Input: part model. Units: mm. Frame: model coordinates. A direction names the side the tool comes from. Coordinates: 2 decimals unless noted, no trailing zeros. Write each loop counter-clockwise with the first axis right and the second up, starting at its lowest first coordinate (ties: lowest second). Pieces come first, ordered by that corner, then holes. Notation, with made-up numbers: M 88.25,89.25 L 131.25,89.25 A36 ccw 131.25,124.25 Z; hole C 36.5,-36 d8. An arc over 180 degrees is marked long. Use CSV: the item, a comma, the result in double quotes.
Autodesk Inventor part; units mm, degrees
ref_plane "YZ Plane" through (0, 0, 0) normal (1, 0, 0) x (0, 1, 0)
ref_plane "XZ Plane" through (0, 0, 0) normal (0, 1, 0) x (-1, 0, 0)
ref_plane "XY Plane" through (0, 0, 0) normal (0, 0, 1) x (1, 0, 0)
sketch "Sketch1" plane through (0, 0, 0) normal (0, 0, 1) x (1, 0, 0)
  arc A0 (20, 0) -> (-20, 0) centre (0, 0) ccw
  line L0 (-20, 0) -> (-20, -104)
  line L1 (20, 0) -> (20, -52)
  arc A1 (19.4895, -54.5451) -> (20, -52) centre (13.4, -52) ccw
  arc A2 (-20, -104) -> (-7.0525, -122.7153) centre (0, -104) ccw
  arc A3 (-7.0525, -122.7153) -> (19.963, -105.2168) centre (0, -104) ccw
  arc A4 (19.963, -105.2168) -> (12.0286, -88.0215) centre (0, -104) ccw
  arc A5 (9.4588, -78.5451) -> (12.0286, -88.0215) centre (16.84, -81.6301) ccw
  line L2 (9.4588, -78.5451) -> (19.4895, -54.5451)
  line L3 (-10, 5.5) -> (10.3, 5.5)
  line L4 (10.3, 5.5) -> (10.3, -35.5)
  line L5 (10.3, -35.5) -> (-10, -35.5)
  line L6 (-10, -35.5) -> (-10, 5.5)
  dimension "d3" = 20
  dimension "d5" = 52
  dimension "d6" = 20
  dimension "d7" = 20
  dimension "d8" = 8
  dimension "d10" = 6.6
  dimension "d11" = 24
  dimension "d17" = 20.3
  dimension "d18" = 41
  dimension "d19" = 10
  dimension "d20" = 104
  dimension "d30" = 5.5
extrude "Extrusion1" add sketch "Sketch1" along normal blind 3.3
sketch "Sketch2" plane through (0, 0, 3.3) normal (0, 0, 1) x (1, 0, 0)
  line L0 (-10, 5.5) -> (10.3, 5.5)
  line L1 (10.3, -35.5) -> (-10, -35.5)
  circle A0 centre (-5, 10) radius 1
  circle A1 centre (-5, -40.25) radius 1
  line L2 (-10, -35.5) -> (-10, 5.5)
  line L3 (10.3, 5.5) -> (10.3, -35.5)
  circle A2 centre (5, 10) radius 1
  circle A3 centre (5, -40.25) radius 1
  point P0 (0, 0)
  dimension "d31" = 2
  dimension "d32" = 2
  dimension "d34" = 4.5
  dimension "d36" = 4.75
  dimension "d65" = 5
  dimension "d66" = 10
  dimension "d67" = 5
  dimension "d68" = 10
extrude "Extrusion2" cut sketch "Sketch2" against normal blind 4.5 contours A0 | A1 | A2 | A3
sketch "Sketch3" plane through (0, 0, 3.3) normal (0, 0, 1) x (1, 0, 0)
  line L0 (-20, 0) -> (-20, -104)
  line L1 (10.3, 5.5) -> (10.3, -35.5)
  line L2 (10.3, -35.5) -> (-10, -35.5)
  line L3 (-10, -35.5) -> (-10, 5.5)
  line L4 (-10, 5.5) -> (10.3, 5.5)
  line L5 (-20, 0) -> (-20, -104)
  arc A0 (-20, -104) -> (12.0286, -88.0215) centre (0, -104) ccw
  arc A1 (9.4588, -78.5451) -> (12.0286, -88.0215) centre (16.84, -81.6301) ccw
  line L6 (9.4588, -78.5451) -> (19.4895, -54.5451)
  arc A2 (19.4895, -54.5451) -> (20, -52) centre (13.4, -52) ccw
  line L7 (20, -52) -> (20, 0)
  arc A3 (20, 0) -> (-20, 0) centre (0, 0) ccw
  line L8 (-15, -86) -> (-15, -56)
  line L9 (15, -45.2979) -> (15, -53.2979)
  line L10 (15, -53.2979) -> (4.448, -78.5451)
  line L11 (4.448, -78.5451) -> (-15, -86)
  line L12 (9.4588, -78.5451) -> (19.4895, -54.5451)
  line L13 (-15, -94.5676) -> (-15, -104)
  arc A4 (-15, -104) -> (9.0215, -92.0161) centre (0, -104) ccw
  arc A5 (-20, -104) -> (12.0286, -88.0215) centre (0, -104) ccw
  arc A6 (4.9629, -86.9153) -> (9.0215, -92.0161) centre (16.84, -81.6301) ccw
  arc A7 (9.4588, -78.5451) -> (12.0286, -88.0215) centre (16.84, -81.6301) ccw
  line L14 (4.9629, -86.9153) -> (-15, -94.5676)
  line L15 (-15, -56) -> (15, -45.2979)
  line L16 (-15, -50.6914) -> (15, -39.9893)
  line L17 (15, -39.9893) -> (15, -36.8041)
  line L18 (15, -36.8041) -> (-15, -47.5062)
  line L19 (-15, -47.5062) -> (-15, -50.6914)
  point P0 (19.8711, -53.2979)
  dimension "d45" = 5
  dimension "d46" = 5
  dimension "d48" = 8
  dimension "d49" = 18
  dimension "d52" = 5
  dimension "d54" = 3
  dimension "d56" = 30
  dimension "d57" = 8
sketch "Sketch4" plane through (0, 0, 3.3) normal (0, 0, 1) x (1, 0, 0)
  line L0 (10.3, 5.5) -> (-10, 5.5)
  line L1 (-3.6, 5.5) -> (3.6, 5.5)
  line L2 (3.6, 5.5) -> (3.6, 10.6)
  line L3 (3.6, 10.6) -> (-3.6, 10.6)
  line L4 (-3.6, 10.6) -> (-3.6, 5.5)
  line L5 (-10, -35.5) -> (-10, 5.5)
  line L6 (10.3, 5.5) -> (10.3, -35.5)
  point P0 (0, 0)
  dimension "d71" = 5.1
  dimension "d72" = 7.2
  dimension "d73" = 6.4
extrude "Extrusion6" cut sketch "Sketch4" against normal blind 10
equation "\"d3\" = radio_muslo"
equation "\"d6\" = radio_muslo"
equation "\"d7\" = d6"
equation "\"d20\" = 2 * d5"
equation "\"d22\" = espesor"
equation "\"d31\" = agujero_servo"
equation "\"d32\" = agujero_servo"
equation "\"d36\" = distancia_agujero_servo"
equation "\"espesor\" = 3.3"
properties part number "Pata - Brazo" material "ABS Plastic"
1. Section C-C (y = -75). Return loops of the section in (x, z).
Resolved:
outline,"M -20,0 L 10.94,0 L 10.94,3.3 L -20,3.3 Z"
2. Access query for faces 1 (the cylindrical face through (19.875, -53.28, 1.627)), 2 (the flat face through (0, 10.6, 2)), 3 (the flat face through (-20, -51, 2)). Directions: +Z, -Z, +X, -X, +Y, -Y. A direction counts if a zero-diameter tool reaches every point of the face in a straight line with its end or side. Return the directions, or none.
Resolved:
face 1,"+Z, -Z, +X"
face 2,"+Z, -Z"
face 3,"+Z, -Z, -X, +Y, -Y"
3. Material intervals for line 1 (Y direction, x = -5, z = 0.9); line 2 (X direction, y = -2, z = 1.5); line 3 (Y direction, x = -3.5, z = 0.75), sorted ascending. Write a range as [from, to].
Resolved:
line 1,"y = [-123.36, -41.25], [-39.25, -35.5], [5.5, 9], [11, 19.36]"
line 2,"x = [-20, -10], [10.3, 20]"
line 3,"y = [-123.69, -35.5], [10.6, 19.69]"
4. Contact query for flat-ended pins moving along their axis: pin 1 Ø1 at (x, z) = (-1.5, 1.5) entering from -Y (3 decimals); pin 2 Ø1 at (y, z) = (-75.5, 2.5) entering from +X; pin 3 Ø1.6 at (y, z) = (8, 2.5) entering from +X. Output: stop coordinate, or through.
Resolved:
pin 1,"stops at y = -123.975"
pin 2,"stops at x = 10.94"
pin 3,"stops at x = 18.66"
5. Section B-B (z = 2.2). Return loops of the section in (x, y).
Resolved:
outline,"M -20,-104 A20 ccw -7.05,-122.72 A20 ccw 19.96,-105.22 A20 ccw 12.03,-88.02 A8 cw 9.46,-78.55 L 19.49,-54.55 A6.6 ccw 20,-52 L 20,0 A20 ccw -20,0 Z; hole M -10,-35.5 L 10.3,-35.5 L 10.3,5.5 L 3.6,5.5 L 3.6,10.6 L -3.6,10.6 L -3.6,5.5 L -10,5.5 Z; hole C -5,-40.25 d2; hole C -5,10 d2; hole C 5,-40.25 d2; hole C 5,10 d2"
6. Section A-A (x = 0). Return loops of the section in (y, z), then the cut area to 3 significant figures.
Resolved:
outline,"M -124,0 L -35.5,0 L -35.5,3.3 L -124,3.3 Z; M 10.6,0 L 20,0 L 20,3.3 L 10.6,3.3 Z"
area,"323 mm^2"
7. Mould query, pull axis X, two halves, no side actions, for faces 4 (the flat face through (0, -51, 0)), 5 (the cylindrical face through (-16, -116, 2)), 6 (the flat face through (0, -35.5, 2)). Classes: pulls with the +X half, pulls with the -X half, needs draft (parallel to the pull), parting line crosses it, or undercut.
Resolved:
face 4,"needs draft"
face 5,"pulls with the -X half"
face 6,"undercut"
